from build123d import *

# Parameters (mm, degrees)
SKETCH1_R           = 32.5
SKETCH1_R_2         = 2
BOSS_EXTRUDE1_DEPTH = 26
FILLET1_R           = 3
SKETCH2_R           = 23.5
CUT_EXTRUDE1_DEPTH  = 16
SKETCH3_R           = 9
BOSS_EXTRUDE2_DEPTH = 5
SKETCH4_R           = 7.5
CUT_EXTRUDE2_DEPTH  = 2
SKETCH5_R           = 5
CUT_EXTRUDE3_DEPTH  = 4
FILLET2_R           = 3


with BuildPart() as part:
    # Sketch1 → Boss-Extrude1 (new body)
    with BuildSketch(Plane.XY):
        Circle(SKETCH1_R)
        Circle(SKETCH1_R_2, mode=Mode.SUBTRACT)
    extrude(amount=BOSS_EXTRUDE1_DEPTH)

    # Fillet1
    fillet1_edges = [part.edges().sort_by_distance(p)[0] for p in [
        (-32.5, 0, 0),
        (-32.5, 0, 26),
    ]]
    fillet(fillet1_edges, radius=FILLET1_R)

    # Sketch2 → Cut-Extrude1 (cut)
    with BuildSketch(Plane.XY.offset(26)):
        Circle(SKETCH2_R)
    extrude(amount=-CUT_EXTRUDE1_DEPTH, mode=Mode.SUBTRACT)

    # Sketch3 → Boss-Extrude2 (add)
    with BuildSketch(Plane.XY.offset(10)):
        Circle(SKETCH3_R)
        Polygon((-6.05, -3.492969129), (-6.05, 3.492969129), (0, 6.985938257), (6.05, 3.492969129), (6.05, -3.492969129), (0, -6.985938257), align=None, mode=Mode.SUBTRACT)
    extrude(amount=BOSS_EXTRUDE2_DEPTH)

    # Sketch4 → Cut-Extrude2 (cut)
    with BuildSketch(Plane(origin=(0, 0, 0), x_dir=(-1, 0, 0), z_dir=(0, 0, -1))):
        Circle(SKETCH4_R)
    extrude(amount=-CUT_EXTRUDE2_DEPTH, mode=Mode.SUBTRACT)

    # Sketch5 → Cut-Extrude3 (cut)
    with BuildSketch(Plane(origin=(0, 0, 2), x_dir=(-1, 0, 0), z_dir=(0, 0, -1))):
        Circle(SKETCH5_R)
    extrude(amount=-CUT_EXTRUDE3_DEPTH, mode=Mode.SUBTRACT)

    # Fillet2
    fillet2_edges = [part.edges().sort_by_distance(p)[0] for p in [
        (-9, 0, 10),
    ]]
    fillet(fillet2_edges, radius=FILLET2_R)


solid = part.part
Work out the finished part from the listing and answer in its coordinate system (mm). A direction names the side the tool comes from. Give positions to 0.01 mm unless a question says otherwise; leave off trailing zeros. Write each loop counter-clockwise with the first axis right and the second up, starting at its lowest first coordinate (ties: lowest second). Pieces come first, ordered by that corner, then holes. Notation, with made-up numbers: M -27.75,-8 L -3.75,-8 A12 cw -3.75,10 Z; hole C 71,4.25 d2. An arc over 180 degrees is marked long. Answer as CSV lines item,"result".
Q1. A cutting plane is placed at D-D on z = 24. Write down the section's boundary in (x, y), plus the area to 3 significant figures.
A:
outline,"C 0,0 d64.66; hole C 0,0 d47"
area,"1,550 mm²"
Q2. Given P1, Ø5, axis at y = 24, z = 19.5, coming from the -X side; P2, Ø5, axis at x = 23, y = 22.5, coming from the -Z side; P3, Ø3.5, axis at x = 0, y = 0, coming from the +Z side; P4, Ø6, axis at x = 2.5, z = 18, coming from the +Y side, each flat-ended and moving along its own axis, determine where each tip first touches the part or whether it passes through.
A:
P1,"stops at x = -24.37"
P2,"stops at z = 0.01"
P3,"passes through"
P4,"stops at y = 32.5"
Q3. A cutting plane is placed at C-C on z = 5. Write down the section's boundary in (x, y).
A:
outline,"C 0,0 d65; hole C 0,0 d10"
Q4. The mould has two halves that part along Y. Classify faces 1 (the flat face through (6, -6, 0)), 2 (the cylindrical face through (31, 9.76, 12.86)), 3 (the flat face through (-3.067, 5.215, 12.465)): +Y half, -Y half, draft (parallel to the pull), parting line (faces both ways), or undercut.
A:
face 1,"draft"
face 2,"parting line"
face 3,"undercut"
Q5. A cutting plane is placed at B-B on z = 11.5. Write down the section's boundary in (x, y), plus the area to 3 significant figures.
A:
outline,"C 0,0 d65; C 0,0 d18.8; hole C 0,0 d47; hole M -6.05,-3.49 L 0,-6.99 L 6.05,-3.49 L 6.05,3.49 L 0,6.99 L -6.05,3.49 Z"
area,"1,730 mm²"
Q6. Find the intervals of material crossed by probe 1 along Y at (x, z) = (0, 14.75); probe 2 along Y at (x, z) = (0, 3.6); probe 3 along X at (y, z) = (-2, 21.5), in increasing order. Write a range as [from, to].
A:
probe 1,"y = [-32.5, -23.5], [-9, -6.99], [6.99, 9], [23.5, 32.5]"
probe 2,"y = [-32.5, -5], [5, 32.5]"
probe 3,"x = [-32.44, -23.41], [23.41, 32.44]"
Q7. A tool of negligible diameter and unlimited length cuts with its end or side. For faces 4 (the flat face through (-20, -13, 26)), 5 (the flat face through (3.067, -5.215, 12.465)), 6 (the cylindrical face through (1.08, -4.88, 3.97)), from which of +Z, -Z, +X, -X, +Y, -Y can it reach the whole face along a straight path? Write none if from no direction.
A:
face 4,"+Z, +X, -X, +Y, -Y"
face 5,"+Z"
face 6,"-Z"
